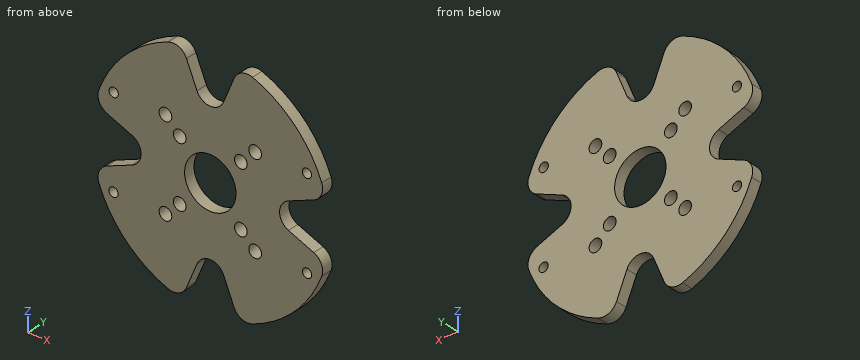
from build123d import *

# Parameters (mm, degrees)
SKETCH1_R                = 41.332242953
SKETCH1_R_2              = 1.6
BOSS_EXTRUDE1_DEPTH      = 4
SKETCH2_R                = 8.913017029
SKETCH2_R_2              = 2.2
CUT_EXTRUDE1_DEPTH       = 12
CUT_EXTRUDE2_START       = -12
CUT_EXTRUDE2_DEPTH       = 12
FILLET1_R                = 5
CIRPATTERN1_COUNT        = 4
FILLET1_OF_CIRPATTERN1_R = 5


with BuildPart() as part:
    # Sketch1 → Boss-Extrude1 (new body)
    with BuildSketch(Plane(origin=(0, 0, 0), x_dir=(1, 0, 0), z_dir=(0, 1, 0))):
        with Locations(Location((-26.014745027, -1.093056514, 0), (0, 0, 270))):
            Circle(SKETCH1_R)
        with Locations(Location((-59.58153309, 14.478552308, 0), (0, 0, 270))):
            Circle(SKETCH1_R_2, mode=Mode.SUBTRACT)
        with Locations(Location((-59.519604899, -16.797470769, 0), (0, 0, 270))):
            Circle(SKETCH1_R_2, mode=Mode.SUBTRACT)
        with Locations(Location((7.490114845, -16.797470769, 0), (0, 0, 270))):
            Circle(SKETCH1_R_2, mode=Mode.SUBTRACT)
        with Locations(Location((7.552043035, 14.478552308, 0), (0, 0, 270))):
            Circle(SKETCH1_R_2, mode=Mode.SUBTRACT)
    extrude(amount=BOSS_EXTRUDE1_DEPTH)

    # Sketch2 → Cut-Extrude1 (cut)
    with BuildSketch(Plane(origin=(0, 4, 0), x_dir=(1, 0, 0), z_dir=(0, 1, 0))):
        with Locations(Location((-26.014745027, -1.093056514, 0), (0, 0, 270))):
            Circle(SKETCH2_R)
        with Locations(Location((-15.408143309, 9.513545204, 0), (0, 0, 270))):
            Circle(SKETCH2_R_2)
        with Locations(Location((-10.458395841, 14.463292672, 0), (0, 0, 270))):
            Circle(SKETCH2_R_2)
        with Locations(Location((-36.621346745, 9.513545204, 0), (0, 0, 270))):
            Circle(SKETCH2_R_2)
        with Locations(Location((-41.571094213, 14.463292672, 0), (0, 0, 270))):
            Circle(SKETCH2_R_2)
        with Locations(Location((-36.621346745, -11.699658232, 0), (0, 0, 270))):
            Circle(SKETCH2_R_2)
        with Locations(Location((-41.571094213, -16.6494057, 0), (0, 0, 270))):
            Circle(SKETCH2_R_2)
        with Locations(Location((-15.408143309, -11.699658232, 0), (0, 0, 270))):
            Circle(SKETCH2_R_2)
        with Locations(Location((-10.458395841, -16.6494057, 0), (0, 0, 270))):
            Circle(SKETCH2_R_2)
    extrude(amount=-CUT_EXTRUDE1_DEPTH, mode=Mode.SUBTRACT)

    # Sketch4 → Cut-Extrude2 (cut)
    with BuildSketch(Plane(origin=(0, 4, 0), x_dir=(1, 0, 0), z_dir=(0, 1, 0)).offset(CUT_EXTRUDE2_START)):
        with BuildLine():
            Line((-66.119037909, 8.906943486), (-41.976902285, -1.093056514))
            Line((-41.976902285, -1.093056514), (-66.119037909, -11.093056514))
            ThreePointArc((-66.119037909, -11.093056514), (-67.34698798, -1.093056514), (-66.119037909, 8.906943486))
        make_face()
    cut_extrude2 = extrude(amount=CUT_EXTRUDE2_DEPTH, mode=Mode.SUBTRACT)

    # Fillet1
    fillet1_edges = [part.edges().sort_by_distance(p)[0] for p in [
        (-66.119037909, 2, 11.093056514),
        (-66.119037909, 2, -8.906943486),
        (-41.976902285, 2, 1.093056514),
    ]]
    fillet(fillet1_edges, radius=FILLET1_R)

    # CirPattern1: Cut-Extrude2 ×4 about axis
    cirpattern1_axis = Axis((-26.014745027, 0, 1.093056514), (0, 1, 0))
    for i in range(1, CIRPATTERN1_COUNT):
        add(cut_extrude2.rotate(cirpattern1_axis, i * 360 / CIRPATTERN1_COUNT), mode=Mode.SUBTRACT)

    # Fillet1 of CirPattern1
    fillet1_of_cirpattern1_edges = [part.edges().sort_by_distance(p)[0] for p in [
        (-16.014745027, 2, 41.197349395),
        (-36.014745027, 2, 41.197349395),
        (-26.014745027, 2, 17.055213772),
        (14.089547854, 2, -8.906943486),
        (14.089547854, 2, 11.093056514),
        (-10.052587769, 2, 1.093056514),
        (-36.014745027, 2, -39.011236368),
        (-16.014745027, 2, -39.011236368),
        (-26.014745027, 2, -14.869100744),
    ]]
    fillet(fillet1_of_cirpattern1_edges, radius=FILLET1_OF_CIRPATTERN1_R)


solid = part.part
The listing builds one solid part. Answer for the finished solid, in the listing's coordinates (mm). Give positions to 0.01 mm unless a question says otherwise; leave off trailing zeros. Write each loop counter-clockwise with the first axis right and the second up, starting at its lowest first coordinate (ties: lowest second). Pieces come first, ordered by that corner, then holes.
Item 1: Section A-A, the plane z = -2.5 is taken. Write down the section's boundary in (x, y), plus the area to 3 significant figures.
Item 2: Section B-B, the plane x = -23.5 is taken. Write down the section's boundary in (y, z), plus the area to 3 significant figures.
Item 3: Section D-D, the plane y = 1.7 is taken. Count the separate pieces of the cut face and the enclosed holes in it, plus the area to 3 significant figures.
Item 4: Find the intervals of material crossed by line 1 along Z through (x, y) = (-36, 2.05); line 2 along Z through (x, y) = (-43, 3.65); line 3 along X through (y, z) = (2.1, -9), in increasing order.
Item 5: Flat-ended cylindrical pins translate along their axes: P1, Ø5, axis at x = -15.41, z = 11.7, coming from the +Y side; P2, Ø2.5, axis at x = -59.58, z = -14.48, coming from the +Y side. Find the tip coordinate at first contact, or state that the pin passes through.
Item 6: Section C-C, the plane z = 11.5 is taken. Write down the section's boundary in (x, y).
Completed:
1. outline: (-51.57, 0) - (-34.17, 0) - (-34.17, 4) - (-51.57, 4) - close; (-17.86, 0) - (-0.46, 0) - (-0.46, 4) - (-17.86, 4) - close
1. area: 139 mm2
2. outline: (0, -23.61) - (4, -23.61) - (4, -7.46) - (0, -7.46) - close; (0, 9.64) - (4, 9.64) - (4, 25.8) - (0, 25.8) - close
2. area: 129 mm2
3. separate pieces: 1
3. enclosed holes: 13
3. area: 4,020 mm2
4. line 1: z = -36.96 to -11.62, -7.4 to 9.59, 13.81 to 39.15
4. line 2: z = -36.59 to -16.14, -12.79 to 14.98, 18.32 to 38.77
4. line 3: x = -64.15 to -38.76, -34.48 to -17.55, -13.27 to 12.12
5. P1: stops at y = 4
5. P2: passes through
6. outline: (-64.34, 0) - (-38.81, 0) - (-38.81, 4) - (-64.34, 4) - close; (-34.43, 0) - (-17.6, 0) - (-17.6, 4) - (-34.43, 4) - close; (-13.22, 0) - (12.31, 0) - (12.31, 4) - (-13.22, 4) - close
